Verification items for the finished model (mm, model axes). Face numbers are marked on the shaded views. Round coordinates to 2 decimals unless told otherwise and drop trailing zeros. Write each loop counter-clockwise with the first axis right and the second up, starting at its lowest first coordinate (ties: lowest second). Pieces come first, ordered by that corner, then holes.
from build123d import *

# Parameters (mm, degrees)
F0_R     = 3.55
F1_DEPTH = 25
F2_SIZE2 = 19.0811366877
F2_SIZE  = 1
F3_R     = 4.5061105162
F4_DEPTH = 15
F5_R     = 2
F6_DEPTH = 25
F7_DEPTH = 8


with BuildPart() as f1:
    # F0 (on Front) → F1 (new body)
    with BuildSketch(Plane.XZ):
        with Locations((-36.0824763775, 37.0747447014)):
            Circle(F0_R)
    extrude(amount=F1_DEPTH)

    # F2
    f2_edges = [f1.edges().sort_by_distance(p)[0] for p in [
        (-39.632476, -25, 37.074745),
    ]]
    f2_side = f1.faces().sort_by_distance((-36.082476, -25, 37.074745))[0]
    chamfer(f2_edges, length=F2_SIZE, length2=F2_SIZE2, reference=f2_side)

    # F3 (on face) → F4 (cut)
    with BuildSketch(Plane.XZ.offset(25)):
        with Locations((-36.0824763775, 37.0747447014)):
            Circle(F3_R)
    extrude(amount=-F4_DEPTH, mode=Mode.SUBTRACT)

    # F5 (on face) → F6 (cut)
    with BuildSketch(Plane.XZ.offset(10)):
        with Locations((-36.0824763775, 37.0747447014)):
            Circle(F5_R)
    extrude(amount=-F6_DEPTH, mode=Mode.SUBTRACT)

    # F7 (add): a face of the model
    f7_faces = [f1.faces().sort_by_distance(p)[0] for p in [
        (-39.5320672146, 0, 37.0747447014),
    ]]
    extrude(f7_faces, amount=F7_DEPTH)


solid = f1.part
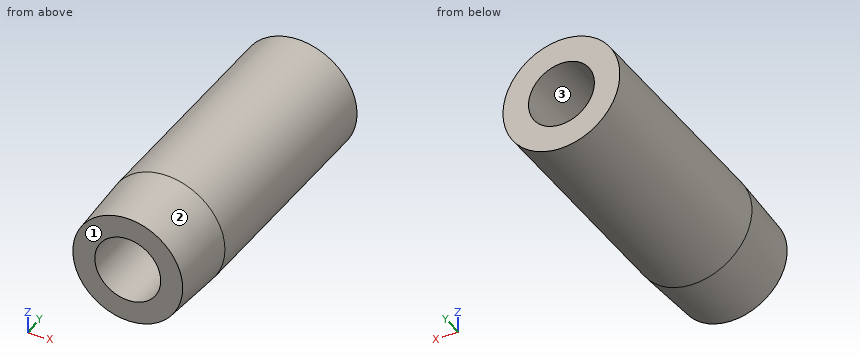
Q1. Material ranges on line 1 along X through (y, z) = (0, 37); line 2 along Z through (x, y) = (-37, 7.25); line 3 along X through (y, z) = (-5.5, 36.25), recorded low to high.
Recorded:
line 1: x = -39.63 to -38.08, -34.08 to -32.53
line 2: z = 33.65 to 35.3, 38.85 to 40.5
line 3: x = -39.54 to -37.9, -34.26 to -32.63
Q2. Depth check by flat-ended pin: P1, Ø2, axis at x = -38.5, y = -7.5, coming from the -Z side. Enter the tip coordinate at first touch or a pass-through.
Recorded:
P1: stops at z = 33.91
Q3. Sectioned sample at B-B (y = -9). Enter the section's corners in (x, z).
Recorded:
outline: circle Ø6.78 at (-36.08, 37.07); hole circle Ø4 at (-36.08, 37.07)
Q4. Sectioned sample at A-A (y = -6.75). Enter the section's corners in (x, z).
Recorded:
outline: circle Ø7.01 at (-36.08, 37.07); hole circle Ø4 at (-36.08, 37.07)
Q5. Release check for a two-part mould opening along X. For the marked faces 1, 2 and 3 record: released by +X, released by -X, zero draft, split by the parting line, or undercut.
Recorded:
face 1: zero draft
face 2: split by the parting line
face 3: undercut
